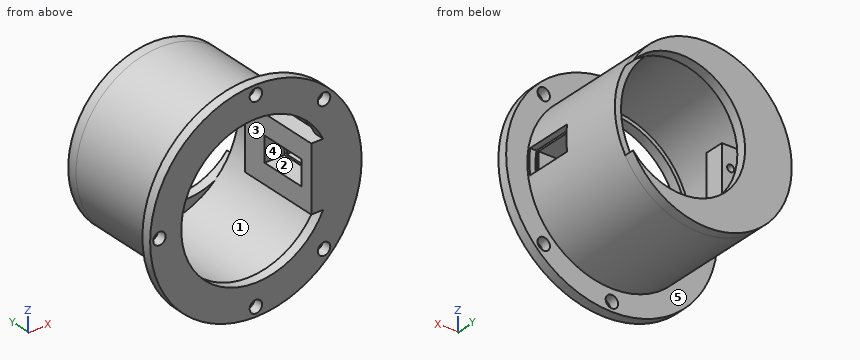
```python
from build123d import *
from build123d.topology import SkipClean

# Parameters (mm, degrees)
SKETCH1_R           = 42.5
SKETCH1_R_2         = 30
BOSS_EXTRUDE1_DEPTH = 4
SKETCH2_R           = 34
SKETCH2_R_2         = 31.5
BOSS_EXTRUDE2_DEPTH = 45
SKETCH3_W           = 8
SKETCH3_H           = 34
SKETCH3_W_2         = 10.5
SKETCH3_H_2         = 8
BOSS_EXTRUDE3_DEPTH = 13
SKETCH4_W           = 10
SKETCH4_H           = 19
CUT_EXTRUDE1_DEPTH  = 92.650490997
SKETCH6_R           = 1.4
CUT_EXTRUDE3_DEPTH  = 7.2
SKETCH8_R           = 2.5
CUT_EXTRUDE4_DEPTH  = 4
BOSS_EXTRUDE4_DEPTH = 4


with BuildPart() as part:
    # Sketch1 → Boss-Extrude1 (new body)
    with BuildSketch(Plane(origin=(0, 0, 0), x_dir=(1, 0, 0), z_dir=(0, 1, 0))):
        with Locations(Location((0, 0, 0), (0, 0, 270))):
            Circle(SKETCH1_R)
        with Locations(Location((0, 0, 0), (0, 0, 270))):
            Circle(SKETCH1_R_2, mode=Mode.SUBTRACT)
    extrude(amount=BOSS_EXTRUDE1_DEPTH)

    # Sketch2 → Boss-Extrude2 (add)
    with BuildSketch(Plane(origin=(0, 4, 0), x_dir=(1, 0, 0), z_dir=(0, 1, 0))):
        with Locations(Location((0, 0, 0), (0, 0, 90))):
            Circle(SKETCH2_R)
        with Locations(Location((0, 0, 0), (0, 0, 90))):
            Circle(SKETCH2_R_2, mode=Mode.SUBTRACT)
    extrude(amount=BOSS_EXTRUDE2_DEPTH)

    # Sketch3 → Boss-Extrude3 (add, symmetric)
    with BuildSketch(Plane.XY):
        with Locations((26.25, 17)):
            Rectangle(SKETCH3_W, SKETCH3_H)
        with Locations((-26, 30)):
            Rectangle(SKETCH3_W_2, SKETCH3_H_2)
    extrude(amount=BOSS_EXTRUDE3_DEPTH, both=True)

    # Sketch4 → Cut-Extrude1 (cut, through all)
    with BuildSketch(Plane.ZY.offset(-22.25)):
        with Locations((0, 14.5)):
            Rectangle(SKETCH4_W, SKETCH4_H)
    extrude(amount=-CUT_EXTRUDE1_DEPTH, mode=Mode.SUBTRACT)

    # Sketch6 → Cut-Extrude3 (cut)
    with BuildSketch(Plane(origin=(0, 34, 0), x_dir=(1, 0, 0), z_dir=(0, 1, 0))):
        with Locations(Location((-24.25, -5, 0), (0, 0, 270))):
            Circle(SKETCH6_R)
        with Locations(Location((24.75, -5, 0), (0, 0, 270))):
            Circle(SKETCH6_R)
        with Locations(Location((24.75, 5, 0), (0, 0, 90))):
            Circle(SKETCH6_R)
        with Locations(Location((-24.25, 5, 0), (0, 0, 90))):
            Circle(SKETCH6_R)
    extrude(amount=-CUT_EXTRUDE3_DEPTH, mode=Mode.SUBTRACT)

    # Sketch8 → Cut-Extrude4 (cut)
    with BuildSketch(Plane(origin=(0, 4, 0), x_dir=(1, 0, 0), z_dir=(0, 1, 0))):
        with Locations(Location((-38.75, 0, 0), (0, 0, 270))):
            Circle(SKETCH8_R)
        with Locations(Location((0, 38.75, 0), (0, 0, 270))):
            Circle(SKETCH8_R)
        with Locations(Location((0, -38.75, 0), (0, 0, 270))):
            Circle(SKETCH8_R)
        with Locations(Location((27.400387771, -27.400387771, 0), (0, 0, 270))):
            Circle(SKETCH8_R)
        with Locations(Location((27.400387771, 27.400387771, 0), (0, 0, 270))):
            Circle(SKETCH8_R)
    extrude(amount=-CUT_EXTRUDE4_DEPTH, mode=Mode.SUBTRACT)

    # Sketch9 → Boss-Extrude4 (add)
    with SkipClean():  # the faces are left unmerged after this step: merging them gives an invalid solid
        with BuildSketch(Plane(origin=(0, 49, 0), x_dir=(1, 0, 0), z_dir=(0, 1, 0))):
            with BuildLine():
                ThreePointArc((29.795731707, 16.377251663), (-15.25, 0), (29.795731707, -16.377251663))
                ThreePointArc((29.795731707, -16.377251663), (-34, 0), (29.795731707, 16.377251663))
            make_face()
        extrude(amount=BOSS_EXTRUDE4_DEPTH)


solid = part.part
```
Work out the finished part from the listing and answer in its coordinate system (mm). Face numbers are marked on the shaded views. A direction names the side the tool comes from. Round coordinates to 2 decimals unless told otherwise and drop trailing zeros. Loops run counter-clockwise (first coordinate to the right, second up) from the corner with the lowest first, then second, coordinate; pieces in that order, holes last. Notation, with made-up numbers: (60.25, 67) -> (118.25, 67) arc R18 ccw to (118.25, 80) -> close; hole circle Ø11 at (0.5, 19). An arc over 180 degrees is marked (long way). Write each question's results on one line, items separated by ' | '. Start each with the question number.
1. Section D-D (z = 0) is taken. State how many separate pieces and enclosed holes the cut face has, plus the area to 4 significant figures.
2. Section C-C (x = -27.5) is taken. Determine the outline of the cut face in (y, z).
3. Section B-B (z = 38.75) is taken. Determine the outline of the cut face in (x, y).
4. Given pin 1 Ø1 at (y, z) = (38.5, -27) entering from +X; pin 2 Ø13 at (y, z) = (16, -5.5) entering from -X; pin 3 Ø4.5 at (x, z) = (24.75, 5) entering from -Y; pin 4 Ø5 at (x, z) = (-33.5, -20.5) entering from +Y, each flat-ended and moving along its own axis, determine where each tip first touches the part or whether it passes through.
5. For a pull along X with two mould halves and no side action, classify the marked faces 1 and 2 as +X half, -X half, draft (parallel to the pull), parting line (faces both ways), or undercut.
6. Find the intervals of material crossed by probe 1 along Y at (x, z) = (5, 30); probe 2 along Y at (x, z) = (-14.5, 38.5); probe 3 along Z at (x, y) = (-2, 7.5), in increasing order. Write a range as from..to.
7. A tool of negligible diameter and unlimited length cuts with its end or side. For the marked faces 3, 4 and 5, from which of +Z, -Z, +X, -X, +Y, -Y can it reach the whole face along a straight path? Write none if from no direction.
8. Section A-A (y = 31) is taken. Determine the outline of the cut face in (x, z).
Evaluation:
1) separate pieces: 6 | enclosed holes: 0 | area: 535.5 mm2
2) outline: (0, -32.4) -> (4, -32.4) -> (4, -19.99) -> (53, -19.99) -> (53, 19.99) -> (4, 19.99) -> (4, 32.4) -> (0, 32.4) -> (0, 11.99) -> (4, 11.99) -> (4, 15.36) -> (49, 15.36) -> (49, -15.36) -> (4, -15.36) -> (4, -11.99) -> (0, -11.99) -> close; (26, -13) -> (34, -13) -> (34, 13) -> (26, 13) -> close
3) outline: (-17.46, 0) -> (-2.5, 0) -> (-2.5, 4) -> (-17.46, 4) -> close; (2.5, 0) -> (17.46, 0) -> (17.46, 4) -> (2.5, 4) -> close
4) pin 1: stops at x = 21.3 | pin 2: stops at x = -34 | pin 3: stops at y = 0 | pin 4: stops at y = 4
5) face 1: undercut | face 2: draft
6) probe 1: y = 0..4, 49..53 | probe 2: y = 0..4 | probe 3: z = -33.94..-31.44, 31.44..33.94
7) face 3: +Y, -Y | face 4: +X | face 5: +Y
8) outline: circle Ø68 at (0, 0); hole (-31.25, -3.96) -> (-31.25, 3.96) arc R31.5 ccw to start; hole (-28.69, -13) arc R31.5 ccw to (28.69, -13) -> (22.25, -13) -> (22.25, 13) -> (28.69, 13) arc R31.5 ccw to (-28.69, 13) -> (-20.75, 13) -> (-20.75, -13) -> close; hole circle Ø2.8 at (-24.25, -5); hole circle Ø2.8 at (-24.25, 5); hole circle Ø2.8 at (24.75, -5); hole circle Ø2.8 at (24.75, 5); hole (30.25, -8.79) arc R31.5 ccw to (30.25, 8.79) -> close
